Autodesk Fusion 360 part; units mm, degrees
sketch "Sketch1" plane through (0, 0, 0) normal (1, 0, 0) x (0, 0, -1)
  circle A0 centre (0, 0) radius 6
  circle A1 centre (0, 0) radius 9
  dimension "d1" = 12
  dimension "d2" = 18
extrude "Extrude1" add sketch "Sketch1" along normal blind 12 makes body 1
copy_body "Body->Comp1" bodies 1 removing the originals makes body 2 in component "12x18x12 bushing"
component "12x18x12 bushing" placed x (1, 0, 0) y (0, 1, 0) z (0, 0, 1) at (0, 0, 0)
The model under review builds one solid part; all positions refer to its coordinate system, in mm. Coordinates: 2 decimals unless noted, no trailing zeros. Write each loop counter-clockwise with the first axis right and the second up, starting at its lowest first coordinate (ties: lowest second). Pieces come first, ordered by that corner, then holes. Notation, with made-up numbers: (-32.75, -28.5) - (6.25, -28.5) arc R24 ccw to (6.25, -1.5) - close; hole circle Ø7 at (3, 11). An arc over 180 degrees is marked (long way). Write item = value, one per line.
(1) Consider section C-C, the plane x = 7. Give the boundary of the cut face in (y, z), then the cut area to 3 significant figures.
Result sheet:
outline = circle Ø18 at (0, 0); hole circle Ø12 at (0, 0)
area = 141 mm^2
(2) Consider section D-D, the plane y = -6.5. Give the boundary of the cut face in (x, z).
Result sheet:
outline = (0, -6.22) - (12, -6.22) - (12, 6.22) - (0, 6.22) - close
(3) For P1, Ø4, axis at x = 7.5, y = -2, coming from the +Z side; P2, Ø1, axis at x = 3.5, z = 2, coming from the +Y side; P3, Ø2, axis at x = 3, z = -7, coming from the +Y side; P4, Ø4, axis at x = 9, z = -6, coming from the +Y side, all flat-tipped, find the tip position at first contact; note any pin that passes through.
Result sheet:
P1 = 9
P2 = 8.87
P3 = 6.71
P4 = 8.06
(4) Mouldability with a two-part tool opening along Z and no side actions: class faces 1 (the face through (6, 0, 6)), 2 (the face through (0, -6, -2)), 3 (the face through (5.916, -8.923, 1.172)) as pulls with the +Z half, pulls with the -Z half, needs draft (parallel to the pull), parting line crosses it, or undercut.
Result sheet:
face_1 = undercut
face_2 = needs draft
face_3 = parting line crosses it
(5) For line 1 (Y direction, x = 7.25, z = 0); line 2 (Y direction, x = 4.25, z = -1.25); line 3 (Z direction, x = 11, y = -4.25), list the stretches that pass through material, from the lowest coordinate up. Write a range as [from, to].
Result sheet:
line_1 = [-9, -6], [6, 9]
line_2 = [-8.91, -5.87], [5.87, 8.91]
line_3 = [-7.93, -4.24], [4.24, 7.93]
(6) Consider section A-A, the plane y = 0. Give the boundary of the cut face in (x, z).
Result sheet:
outline = (0, -9) - (12, -9) - (12, -6) - (0, -6) - close; (0, 6) - (12, 6) - (12, 9) - (0, 9) - close
